```python
from build123d import *

# Parameters (mm, degrees)
SKETCH_1_W          = 25
SKETCH_1_H          = 5
SKETCH_1_W_2        = 70
SKETCH_1_H_2        = 190
EXTRUDE_1_DEPTH     = 5
SKETCH_2_R          = 1.55
CUT_EXTRUDE_1_DEPTH = 5
SKETCH_3_W          = 50
SKETCH_3_H          = 72.5
CUT_EXTRUDE_2_DEPTH = 5
FILLET_1_R          = 10
FILLET_2_R          = 1
MOVE_FACE_1_BY      = 0.05
MOVE_FACE_1_2_BY    = 0.05
MOVE_FACE_1_3_BY    = 0.05
MOVE_FACE_1_4_BY    = 0.05
MOVE_FACE_1_5_BY    = 0.05
MOVE_FACE_1_6_BY    = 0.05
MOVE_FACE_1_7_BY    = 0.05
MOVE_FACE_1_8_BY    = 0.05
MOVE_FACE_1_9_BY    = 0.05
MOVE_FACE_1_10_BY   = 0.05
MOVE_FACE_1_11_BY   = 0.05
MOVE_FACE_1_12_BY   = 0.05
MOVE_FACE_1_13_BY   = 0.05
MOVE_FACE_1_14_BY   = 0.05
MOVE_FACE_1_15_BY   = 0.05
MOVE_FACE_1_16_BY   = 0.05
MOVE_FACE_1_17_BY   = 0.05
MOVE_FACE_1_18_BY   = 0.05
MOVE_FACE_1_19_BY   = 0.05
MOVE_FACE_1_20_BY   = 0.05


with BuildPart() as part:
    # 草图1 → 凸台-拉伸1 (new body)
    with BuildSketch(Plane.XY):
        with Locations((57.5, 192.5)):
            Rectangle(SKETCH_1_W, SKETCH_1_H)
        with Locations((35, 95)):
            Rectangle(SKETCH_1_W_2, SKETCH_1_H_2)
        with Locations((12.5, 192.5)):
            Rectangle(SKETCH_1_W, SKETCH_1_H)
        with Locations((57.5, -2.5)):
            Rectangle(SKETCH_1_W, SKETCH_1_H)
        with Locations((12.5, -2.5)):
            Rectangle(SKETCH_1_W, SKETCH_1_H)
    extrude(amount=EXTRUDE_1_DEPTH)

    # 草图2 → 切除-拉伸1 (cut)
    with BuildSketch(Plane.XY.offset(5)):
        with Locations((43.45, 0)):
            Circle(SKETCH_2_R)
        with Locations((26.55, 0)):
            Circle(SKETCH_2_R)
        with Locations((43.45, 190)):
            Circle(SKETCH_2_R)
        with Locations((26.55, 190)):
            Circle(SKETCH_2_R)
    extrude(amount=-CUT_EXTRUDE_1_DEPTH, mode=Mode.SUBTRACT)

    # 草图3 → 切除-拉伸2 (cut)
    with BuildSketch(Plane.XY.offset(5)):
        with Locations((35, 51.25)):
            Rectangle(SKETCH_3_W, SKETCH_3_H)
        with Locations((35, 138.75)):
            Rectangle(SKETCH_3_W, SKETCH_3_H)
    extrude(amount=-CUT_EXTRUDE_2_DEPTH, mode=Mode.SUBTRACT)

    # 圆角1
    fillet_1_edges = [part.edges().sort_by_distance(p)[0] for p in [
        (10, 175, 2.5),
        (60, 175, 2.5),
        (60, 102.5, 2.5),
        (10, 15, 2.5),
        (10, 87.5, 2.5),
        (60, 87.5, 2.5),
        (60, 15, 2.5),
        (10, 102.5, 2.5),
    ]]
    fillet(fillet_1_edges, radius=FILLET_1_R)

    # 圆角2
    fillet_2_edges = [part.edges().sort_by_distance(p)[0] for p in [
        (45, 195, 2.5),
        (70, 195, 2.5),
        (70, -5, 2.5),
        (0, -5, 2.5),
        (0, 195, 2.5),
        (25, 195, 2.5),
    ]]
    fillet(fillet_2_edges, radius=FILLET_2_R)

    # Move Face 1: a curved face moved inward by 0.05
    add(Solid.thicken(part.faces().sort_by_distance((69.707106781, -4.707106781, 2.5))[0], -MOVE_FACE_1_BY), mode=Mode.SUBTRACT)

    # Move Face 1 2: a face moved inward by 0.05
    extrude(part.faces().sort_by_distance((57, -5, 2.5))[0], amount=MOVE_FACE_1_2_BY, dir=(0, 1, 0), mode=Mode.SUBTRACT)

    # Move Face 1 3: a face moved inward by 0.05
    extrude(part.faces().sort_by_distance((45, -2.5, 2.5))[0], amount=MOVE_FACE_1_3_BY, dir=(1, 0, 0), mode=Mode.SUBTRACT)

    # Move Face 1 4: a curved face moved inward by 0.05
    add(Solid.thicken(part.faces().sort_by_distance((43.45, 1.55, 2.5))[0], -MOVE_FACE_1_4_BY), mode=Mode.SUBTRACT)

    # Move Face 1 5: a face moved inward by 0.05
    extrude(part.faces().sort_by_distance((25, -2.5, 2.5))[0], amount=MOVE_FACE_1_5_BY, dir=(-1, 0, 0), mode=Mode.SUBTRACT)

    # Move Face 1 6: a curved face moved inward by 0.05
    add(Solid.thicken(part.faces().sort_by_distance((26.55, 1.55, 2.5))[0], -MOVE_FACE_1_6_BY), mode=Mode.SUBTRACT)

    # Move Face 1 7: a face moved inward by 0.05
    extrude(part.faces().sort_by_distance((13, -5, 2.5))[0], amount=MOVE_FACE_1_7_BY, dir=(0, 1, 0), mode=Mode.SUBTRACT)

    # Move Face 1 8: a curved face moved inward by 0.05
    add(Solid.thicken(part.faces().sort_by_distance((0.292893219, -4.707106781, 2.5))[0], -MOVE_FACE_1_8_BY), mode=Mode.SUBTRACT)

    # Move Face 1 9: a face moved inward by 0.05
    extrude(part.faces().sort_by_distance((0, 95, 2.5))[0], amount=MOVE_FACE_1_9_BY, dir=(1, 0, 0), mode=Mode.SUBTRACT)

    # Move Face 1 10: a curved face moved inward by 0.05
    add(Solid.thicken(part.faces().sort_by_distance((0.292893219, 194.707106781, 2.5))[0], -MOVE_FACE_1_10_BY), mode=Mode.SUBTRACT)

    # Move Face 1 11: a face moved inward by 0.05
    extrude(part.faces().sort_by_distance((12.5, 195, 2.5))[0], amount=MOVE_FACE_1_11_BY, dir=(0, -1, 0), mode=Mode.SUBTRACT)

    # Move Face 1 12: a curved face moved inward by 0.05
    add(Solid.thicken(part.faces().sort_by_distance((24.707106781, 194.707106781, 2.5))[0], -MOVE_FACE_1_12_BY), mode=Mode.SUBTRACT)

    # Move Face 1 13: a face moved inward by 0.05
    extrude(part.faces().sort_by_distance((25, 192, 2.5))[0], amount=MOVE_FACE_1_13_BY, dir=(-1, 0, 0), mode=Mode.SUBTRACT)

    # Move Face 1 14: a curved face moved inward by 0.05
    add(Solid.thicken(part.faces().sort_by_distance((26.55, 188.45, 2.5))[0], -MOVE_FACE_1_14_BY), mode=Mode.SUBTRACT)

    # Move Face 1 15: a curved face moved inward by 0.05
    add(Solid.thicken(part.faces().sort_by_distance((43.45, 188.45, 2.5))[0], -MOVE_FACE_1_15_BY), mode=Mode.SUBTRACT)

    # Move Face 1 16: a face moved inward by 0.05
    extrude(part.faces().sort_by_distance((45, 192, 2.5))[0], amount=MOVE_FACE_1_16_BY, dir=(1, 0, 0), mode=Mode.SUBTRACT)

    # Move Face 1 17: a curved face moved inward by 0.05
    add(Solid.thicken(part.faces().sort_by_distance((45.292893219, 194.707106781, 2.5))[0], -MOVE_FACE_1_17_BY), mode=Mode.SUBTRACT)

    # Move Face 1 18: a face moved inward by 0.05
    extrude(part.faces().sort_by_distance((57.5, 195, 2.5))[0], amount=MOVE_FACE_1_18_BY, dir=(0, -1, 0), mode=Mode.SUBTRACT)

    # Move Face 1 19: a curved face moved inward by 0.05
    add(Solid.thicken(part.faces().sort_by_distance((69.707106781, 194.707106781, 2.5))[0], -MOVE_FACE_1_19_BY), mode=Mode.SUBTRACT)

    # Move Face 1 20: a face moved inward by 0.05
    extrude(part.faces().sort_by_distance((70, 95, 2.5))[0], amount=MOVE_FACE_1_20_BY, dir=(-1, 0, 0), mode=Mode.SUBTRACT)


solid = part.part
```
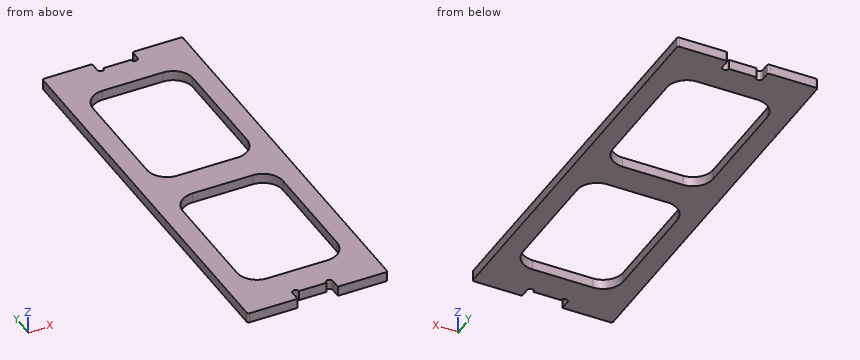
CAD build for the part. Positions are in the model's coordinates, mm. Give positions to 0.01 mm unless a question says otherwise; leave off trailing zeros. Order: outer loops, then holes, each group sorted by start corner. A loop starts at its lowest first (then second) coordinate and runs counter-clockwise, first axis right, second up.
(1) Saw through at B-B, the plane x = 35. Give the cut face in (y, z).
(2) Saw through at A-A, the plane y = 35.5. Give the cut face in (x, z), then the cut area to 3 significant figures.
(3) Drill centre lines: L1, parallel to Y at x = 39, z = 4.6; L2, parallel to X at y = 56.5, z = 1.25; L3, parallel to Y at x = 22, z = 3.6. Where is each one in solid material? Low to high.
(4) Saw through at C-C, the plane z = 2.9. State how many separate pieces and enclosed holes the cut face has, then the cut area to 3 significant figures.
(5) Flat gauge pins, fed straight in: pin 1 (2.5 mm diameter, centred on x = 40.5, z = 2, fed in from +Y); pin 2 (1.5 mm diameter, centred on x = 29, z = 3.5, fed in from -Y); pin 3 (6 mm diameter, centred on x = 32.5, y = 95.5, fed in from -Z). Where does each tip first touch, or does it go through?
(6) Saw through at D-D, the plane y = 84. Give the cut face in (x, z).
Results found:
1. outline: (0, 0) - (15, 0) - (15, 5) - (0, 5) - close; (87.5, 0) - (102.5, 0) - (102.5, 5) - (87.5, 5) - close; (175, 0) - (190, 0) - (190, 5) - (175, 5) - close
2. outline: (0.05, 0) - (10, 0) - (10, 5) - (0.05, 5) - close; (60, 0) - (69.95, 0) - (69.95, 5) - (60, 5) - close
2. area: 99.5 mm2
3. L1: y = 0 to 15, 87.5 to 102.5, 175 to 190
3. L2: x = 0.05 to 10, 60 to 69.95
3. L3: y = -4.95 to 15, 87.5 to 102.5, 175 to 194.95
4. separate pieces: 1
4. enclosed holes: 2
4. area: 6,680 mm2
5. pin 1: stops at y = 190
5. pin 2: stops at y = 0
5. pin 3: stops at z = 0
6. outline: (0.05, 0) - (12.4, 0) - (12.4, 5) - (0.05, 5) - close; (57.6, 0) - (69.95, 0) - (69.95, 5) - (57.6, 5) - close
